Can you work these out from the model? Positions are in its coordinate system, mm. Face numbers are marked on the shaded views. A direction names the side the tool comes from. Coordinates: 2 decimals unless noted, no trailing zeros. Order: outer loops, then holes, each group sorted by start corner. A loop starts at its lowest first (then second) coordinate and runs counter-clockwise, first axis right, second up. Notation, with made-up numbers: (-3.75, -7.75) - (44.25, -7.75) arc R20 cw to (44.25, 11.25) - close; hole circle Ø7 at (-2, 68.25). An arc over 180 degrees is marked (long way). Use a Markdown table: item, result. Add a question column.
(1) I want a section at C-C (z = 5.5). List the corners of the cut face in (x, y) for me, and give its area (3 significant figures).
(2) I want a section at A-A (y = 10). List the corners of the cut face in (x, z) for me.
(3) We'd pull the mould along X, two halves only. Please class the marked faces 4, 5, 6 and 7: pulls with the +X half, pulls with the -X half, needs draft (parallel to the pull), parting line crosses it, or undercut.
(4) If I drill on L1, parallel to Y at x = 1, z = 3.75; L2, parallel to Y at x = 5.25, z = 2.5; L3, parallel to Z at x = 3.25, y = -22.5, over which ranges is the centre line in solid material (lowest first)? Write a range as [from, to].
(5) For pin 1 Ø0.8 at (x, z) = (-2.5, 6) entering from +Y; pin 2 Ø1.7 at (x, z) = (-1.5, 2.5) entering from +Y; pin 3 Ø1.7 at (x, z) = (10, 5.5) entering from -Y, each with a flat end and sliding along its axis, tell me the tip position at first contact or that it passes through.
(6) I want a section at D-D (z = 7.25). List the corners of the cut face in (x, y) for me, and give its area (3 significant figures).
(7) On a 3-axis mill with a long thin cutter (end or side, diameter ignored), from which of +Z, -Z, +X, -X, +Y, -Y can I reach the whole of each face in a straight line? I mean the marked faces 1, 2 and 3. Say none if no direction works.
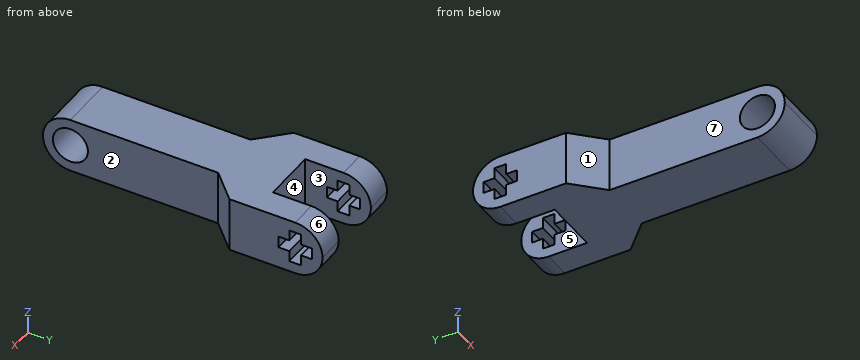
```python
from build123d import *

# Parameters (mm, degrees)
F0_W     = 7.9375
F0_H     = 25.4
F1_DEPTH = 7.9375
F2_R     = 3.96874
F3_W     = 1.6891
F3_H     = 1.56845
F3_W_2   = 1.56845
F3_H_2   = 1.6891
F3_R     = 2.54
F4_DEPTH = 15.875


# Not quite as in the source:
# - a fillet or chamfer is up to 0.001 mm smaller than in the source, because OpenCascade refuses the exact size


with BuildPart() as f1:
    # F0 (on Top) → F1 (new body)
    with BuildSketch(Plane.XY):
        Polygon((-3.96875, 3.96875), (0, 0), (7.9375, 0), (11.90625, 3.96875), (11.90625, 17.4625), (7.9375, 17.4625), (7.9375, 7.9375), (0, 7.9375), (0, 17.4625), (-3.96875, 17.4625), align=None)
        with Locations((3.96875, -12.7)):
            Rectangle(F0_W, F0_H)
    extrude(amount=F1_DEPTH)

    # F2 (radius 3.96875 in the source; OpenCascade refuses exactly that, so slightly less here)
    f2_edges = [f1.edges().sort_by_distance(p)[0] for p in [
        (3.96875, -25.4, 7.9375),
        (3.96875, -25.4, 0),
        (9.921875, 17.4625, 7.9375),
        (9.921875, 17.4625, 0),
        (-1.984375, 17.4625, 7.9375),
        (-1.984375, 17.4625, 0),
    ]]
    fillet(f2_edges, radius=F2_R)

    # F3 (on face) → F4 (cut, through all)
    with BuildSketch(Plane.YZ.offset(11.90625)):
        with Locations((13.49375, 5.597525)):
            Rectangle(F3_W, F3_H)
        with Locations((15.122525, 3.96875)):
            Rectangle(F3_W_2, F3_H_2)
        with Locations((13.49375, 3.96875)):
            Rectangle(F3_W, F3_H_2)
        with Locations((11.864975, 3.96875)):
            Rectangle(F3_W_2, F3_H_2)
        with Locations((13.49375, 2.339975)):
            Rectangle(F3_W, F3_H)
        with Locations((-21.43125, 3.96875)):
            Circle(F3_R)
    extrude(amount=-F4_DEPTH, mode=Mode.SUBTRACT)


solid = f1.part
```
Answers follow:
| question | item | result |
|---|---|---|
| 1 | outline | (-3.97, 3.97) - (0, 0) - (0, -19.4) - (7.94, -19.4) - (7.94, 0) - (11.91, 3.97) - (11.91, 12.65) - (7.94, 12.65) - (7.94, 7.94) - (0, 7.94) - (0, 12.65) - (-3.97, 12.65) - close; (-3.97, 14.34) - (0, 14.34) - (0, 17.16) - (-3.97, 17.16) - close; (0, -25.09) - (7.94, -25.09) - (7.94, -23.46) - (0, -23.46) - close; (7.94, 14.34) - (11.91, 14.34) - (11.91, 17.16) - (7.94, 17.16) - close |
| 1 | area | 337 mm² |
| 2 | outline | (-3.97, 0) - (0, 0) - (0, 7.94) - (-3.97, 7.94) - close; (7.94, 0) - (11.91, 0) - (11.91, 7.94) - (7.94, 7.94) - close |
| 3 | face 4 | undercut |
| 3 | face 5 | undercut |
| 3 | face 6 | needs draft |
| 3 | face 7 | pulls with the -X half |
| 4 | L1 | y = [-25.39, -23.96], [-18.9, 7.94] |
| 4 | L2 | y = [-25.12, -23.5], [-19.36, 7.94] |
| 4 | L3 | z = [0.15, 1.66], [6.27, 7.79] |
| 5 | pin 1 | stops at y = 17.11 |
| 5 | pin 2 | stops at y = 17.41 |
| 5 | pin 3 | stops at y = 1.21 |
| 6 | outline | (-3.97, 3.97) - (0, 0) - (0, -23.66) - (7.94, -23.66) - (7.94, 0) - (11.91, 3.97) - (11.91, 15.73) - (7.94, 15.73) - (7.94, 7.94) - (0, 7.94) - (0, 15.73) - (-3.97, 15.73) - close |
| 6 | area | 360 mm² |
| 7 | face 1 | +Z, -Z, -X, -Y |
| 7 | face 2 | +Z, -Z, +X, -Y |
| 7 | face 3 | +Z, -Z, +Y |
